from build123d import *

# Parameters (mm, degrees)
SKETCH3_W            = 42.8
SKETCH3_H            = 40
BOSS_EXTRUDE1_DEPTH  = 6.35
SKETCH4_R            = 12.4
CUT_EXTRUDE1_DEPTH   = 12.8
SKETCH5_R            = 12.115
CUT_EXTRUDE2_DEPTH   = 31
SKETCH6_W            = 8
SKETCH6_H            = 4
BOSS_EXTRUDE2_DEPTH  = 53.2
SKETCH7_R            = 2.25
CUT_EXTRUDE3_DEPTH   = 4
LPATTERN1_COUNT      = 3
LPATTERN1_PITCH      = 16
LPATTERN1_COUNT_DIR2 = 2
LPATTERN1_PITCH_DIR2 = 32


with BuildPart() as part:
    # Sketch3 → Boss-Extrude1 (new body)
    with BuildSketch(Plane(origin=(0, 0, 0), x_dir=(1, 0, 0), z_dir=(0, 1, 0))):
        with Locations((48, 0)):
            Rectangle(SKETCH3_W, SKETCH3_H)
        with BuildLine():
            Line((32, 18.4), (64, 18.4))
            ThreePointArc((64, 18.4), (66.4, 16), (64, 13.6))
            Line((64, 13.6), (32, 13.6))
            ThreePointArc((32, 13.6), (29.6, 16), (32, 18.4))
        make_face(mode=Mode.SUBTRACT)
        with BuildLine():
            Line((32, -18.4), (64, -18.4))
            ThreePointArc((64, -18.4), (66.4, -16), (64, -13.6))
            Line((64, -13.6), (32, -13.6))
            ThreePointArc((32, -13.6), (29.6, -16), (32, -18.4))
        make_face(mode=Mode.SUBTRACT)
    extrude(amount=BOSS_EXTRUDE1_DEPTH)

    # Sketch4 → Cut-Extrude1 (cut)
    with BuildSketch(Plane(origin=(69.4, 0, 0), x_dir=(0, 0, -1), z_dir=(1, 0, 0))):
        with Locations((0, -7.874)):
            Circle(SKETCH4_R)
    extrude(amount=-CUT_EXTRUDE1_DEPTH, mode=Mode.SUBTRACT)

    # Sketch5 → Cut-Extrude2 (cut, through all)
    with BuildSketch(Plane(origin=(56.6, 0, 0), x_dir=(0, 0, -1), z_dir=(1, 0, 0))):
        with Locations((0, -7.874)):
            Circle(SKETCH5_R)
    extrude(amount=-CUT_EXTRUDE2_DEPTH, mode=Mode.SUBTRACT)


with BuildPart() as body_2:
    # Mirror2: mirrored copy
    add(part.part.mirror(Plane(origin=(0, 0, 0), x_dir=(0, 0, 1), z_dir=(1, 0, 0))))


with BuildPart() as part_1:
    add(part.part)

    add(body_2.part)  # Boss-Extrude2 merges body 2
    # Sketch6 → Boss-Extrude2 (add)
    with BuildSketch(Plane.ZY.offset(-26.6)):
        with Locations((-16, 4.35)):
            Rectangle(SKETCH6_W, SKETCH6_H)
        with Locations((16, 4.35)):
            Rectangle(SKETCH6_W, SKETCH6_H)
    extrude(amount=BOSS_EXTRUDE2_DEPTH)

    # Sketch7 → Cut-Extrude3 (cut)
    with BuildSketch(Plane(origin=(0, 6.35, 0), x_dir=(1, 0, 0), z_dir=(0, 1, 0))):
        with Locations((-16, 16)):
            Circle(SKETCH7_R)
    cut_extrude3 = extrude(amount=-CUT_EXTRUDE3_DEPTH, mode=Mode.SUBTRACT)

    # LPattern1: Cut-Extrude3 3 × 2
    with Locations(*[(i * LPATTERN1_PITCH, 0, j * LPATTERN1_PITCH_DIR2) for i in range(LPATTERN1_COUNT) for j in range(LPATTERN1_COUNT_DIR2) if (i, j) != (0, 0)]):
        add(cut_extrude3, mode=Mode.SUBTRACT)


solid = part_1.part
Geometry check sheet. Reference: the model listing, model coordinates, mm. A direction names the side the tool comes from. Give positions to 0.01 mm unless a question says otherwise; leave off trailing zeros. Loops run counter-clockwise (first coordinate to the right, second up) from the corner with the lowest first, then second, coordinate; pieces in that order, holes last.
(1) Release check for a two-part mould opening along Z. For faces 6 (the flat face through (48, 3, 18.4)), 7 (the flat face through (0, 2.35, 13)), 8 (the flat face through (1, 3, -20)) record: released by +Z, released by -Z, zero draft, split by the parting line, or undercut.
From the geometry:
face 6: undercut
face 7: zero draft
face 8: released by -Z
(2) Section check A-A on x = -44. Record the cut outline in (y, z) (3 decimals).
From the geometry:
outline: (0, -20) - (6.35, -20) - (6.35, -18.4) - (0, -18.4) - close; (0, -13.6) - (6.35, -13.6) - (6.35, 13.6) - (0, 13.6) - (0, 9.207) arc R12.115 cw to (0, -9.207) - close; (0, 18.4) - (6.35, 18.4) - (6.35, 20) - (0, 20) - close
(3) Section check D-D on z = -2.5. Record the cut outline in (x, y).
From the geometry:
outline: (-69.4, 4.27) - (-56.6, 4.27) - (-56.6, 3.98) - (-26.6, 3.98) - (-26.6, 6.35) - (-69.4, 6.35) - close; (26.6, 3.98) - (56.6, 3.98) - (56.6, 4.27) - (69.4, 4.27) - (69.4, 6.35) - (26.6, 6.35) - close
(4) Set-up check for faces 1 (the cylindrical face through (41.81, 4.24, -0.15)), 2 (the cylindrical face through (63.09, 4.525, -0.153)), 3 (the cylindrical face through (-29.6, 3.13, 15.95)), 4 (the flat face through (-48, 0, -13)), 5 (the flat face through (0, 2.35, -19)): record each of +Z, -Z, +X, -X, +Y, -Y from which the full face is reachable in a straight line by a thin tool's end or side.
From the geometry:
face 1: +X, -X, -Y
face 2: +X, -Y
face 3: +Y, -Y
face 4: +Z, -Z, +X, -X, -Y
face 5: +Z, -Z, -Y
(5) Thickness scan on L1, parallel to X at y = 5.15, z = 16; L2, parallel to Z at x = -16, y = 4.3; L3, parallel to X at y = 2.75, z = 6. Record the ranges inside material, lowest first.
From the geometry:
L1: x = -69.4 to -66.4, -29.6 to -18.25, -13.75 to -2.25, 2.25 to 13.75, 18.25 to 29.6, 66.4 to 69.4
L2: z = -20 to -18.25, -13.75 to -12, 12 to 13.75, 18.25 to 20
L3: x = -56.6 to -26.6, 26.6 to 56.6
(6) Depth check by flat-ended pin: pin 1 Ø7 at (x, z) = (-16, 16) entering from +Y; pin 2 Ø5 at (x, z) = (0, -16) entering from -Y; pin 3 Ø1.5 at (x, z) = (52, -2) entering from -Y; pin 4 Ø8 at (x, z) = (45.5, 4.5) entering from -Y. Enter the tip coordinate at first touch or a pass-through.
From the geometry:
pin 1: stops at y = 6.35
pin 2: stops at y = 2.35
pin 3: stops at y = 3.92
pin 4: stops at y = 0.76
(7) Section check B-B on z = -16. Record the cut outline in (x, y), then the cut area to 3 significant figures.
From the geometry:
outline: (-69.4, 0) - (-66.4, 0) - (-66.4, 6.35) - (-69.4, 6.35) - close; (-29.6, 0) - (-26.6, 0) - (-26.6, 2.35) - (-18.25, 2.35) - (-18.25, 6.35) - (-29.6, 6.35) - close; (-13.75, 2.35) - (-2.25, 2.35) - (-2.25, 6.35) - (-13.75, 6.35) - close; (2.25, 2.35) - (13.75, 2.35) - (13.75, 6.35) - (2.25, 6.35) - close; (18.25, 2.35) - (26.6, 2.35) - (26.6, 0) - (29.6, 0) - (29.6, 6.35) - (18.25, 6.35) - close; (66.4, 0) - (69.4, 0) - (69.4, 6.35) - (66.4, 6.35) - close
area: 235 mm2
(8) Section check C-C on x = 0. Record the cut outline in (y, z).
From the geometry:
outline: (2.35, -20) - (6.35, -20) - (6.35, -18.25) - (2.35, -18.25) - close; (2.35, -13.75) - (6.35, -13.75) - (6.35, -12) - (2.35, -12) - close; (2.35, 12) - (6.35, 12) - (6.35, 13.75) - (2.35, 13.75) - close; (2.35, 18.25) - (6.35, 18.25) - (6.35, 20) - (2.35, 20) - close
